from build123d import *

# Parameters (mm, degrees)
F0_W     = 35
F0_H     = 50
F1_DEPTH = 3
F0_W_2   = 38
F0_H_2   = 53
F2_DEPTH = 1.6
F3_DEPTH = 43
F4_R     = 1
F5_W     = 35
F5_H     = 1.5
F6_DEPTH = 41.4


with BuildPart() as f1:
    # F0 (on Top) → F1 (new body)
    with BuildSketch(Plane.XY):
        with Locations((19, 26.5)):
            Rectangle(F0_W, F0_H)
    extrude(amount=-F1_DEPTH)

    # F0 (on Top) → F2 (join)
    with BuildSketch(Plane.XY):
        with Locations((19, 26.5)):
            Rectangle(F0_W_2, F0_H_2)
        with Locations((19, 26.5)):
            Rectangle(F0_W, F0_H, mode=Mode.SUBTRACT)
        with Locations((19, 26.5)):
            Rectangle(F0_W, F0_H)
    extrude(amount=F2_DEPTH)

    # F0 (on Top) → F3 (join)
    with BuildSketch(Plane.XY):
        with Locations((19, 26.5)):
            Rectangle(F0_W_2, F0_H_2)
        with Locations((19, 26.5)):
            Rectangle(F0_W, F0_H, mode=Mode.SUBTRACT)
    extrude(amount=F3_DEPTH)

    # F4
    f4_edges = [f1.edges().sort_by_distance(p)[0] for p in [
        (36.5, 1.5, -1.5),
        (1.5, 1.5, -1.5),
        (1.5, 51.5, -1.5),
        (36.5, 51.5, -1.5),
        (0, 53, 21.5),
        (38, 53, 21.5),
        (0, 0, 21.5),
        (38, 0, 21.5),
    ]]
    fillet(f4_edges, radius=F4_R)

    # F5 (on face) → F6 (join, through all)
    with BuildSketch(Plane.XY.offset(1.6)):
        with Locations((19, 26.5)):
            Rectangle(F5_W, F5_H)
    extrude(amount=F6_DEPTH)


solid = f1.part
Geometry check sheet. Reference: the model listing, model coordinates, mm. A direction names the side the tool comes from. Give positions to 0.01 mm unless a question says otherwise; leave off trailing zeros. Loops run counter-clockwise (first coordinate to the right, second up) from the corner with the lowest first, then second, coordinate; pieces in that order, holes last. Notation, with made-up numbers: M -29.5,7.25 L -18.5,7.25 A19 cw -18.5,19.25 Z; hole C 40.5,6.5 d9. An arc over 180 degrees is marked long. Answer as a JSON object with one key per item and string values. Group by question number.
Item 1: Sectioned sample at C-C on x = 8. Record the boundary of the cut face in (y, z).
Item 2: Sectioned sample at A-A on y = 5.5. Record the boundary of the cut face in (x, z), plus the area to 3 significant figures.
Item 3: Sectioned sample at B-B on z = 24.5. Record the boundary of the cut face in (x, y), plus the area to 3 significant figures.
Item 4: Access from +Z, -Z, +X, -X, +Y, -Y to the whole of each face (thin tool, end or side, straight path). Record for faces 4 (the flat face through (1.5, 26, -1)), 5 (the flat face through (36.5, 39, 22)), 6 (the flat face through (19, 51.5, -1)), 7 (the flat face through (36.5, 26, -1)), 8 (the flat face through (19, 27, 43)).
Item 5: Material ranges on L1, parallel to Y at x = 28, z = 26; L2, parallel to X at y = 38, z = 40.5; L3, parallel to Z at x = 27, y = 36.5, recorded low to high.
Item 6: Mould release check, pull along Y, two halves, no side actions. Record for faces 1 (the flat face through (19, 0, 21)), 2 (the flat face through (19, 25.75, 22)), 3 (the flat face through (1, 27, 0)): pulls with the +Y half, pulls with the -Y half, needs draft (parallel to the pull), parting line crosses it, or undercut.
Item 7: Gauge pin test, flat ends, axial feed: pin 1 (19.5 mm diameter, centred on x = 22.5, y = 37.5, fed in from +Z); pin 2 (1.5 mm diameter, centred on x = 21.5, z = -1, fed in from +Y); pin 3 (2.5 mm diameter, centred on y = 34.5, z = -1.5, fed in from +X). Record the tip position at first contact, or that the pin passes through.
Findings below:
{
 "1": {"outline": "M 0,0 L 1.5,0 L 1.5,-3 L 51.5,-3 L 51.5,0 L 53,0 L 53,43 L 51.5,43 L 51.5,1.6 L 27.25,1.6 L 27.25,43 L 25.75,43 L 25.75,1.6 L 1.5,1.6 L 1.5,43 L 0,43 Z"},
 "2": {"outline": "M 0,0 L 1.5,0 L 1.5,-3 L 36.5,-3 L 36.5,0 L 38,0 L 38,43 L 36.5,43 L 36.5,1.6 L 1.5,1.6 L 1.5,43 L 0,43 Z", "area": "290 mm2"},
 "3": {"outline": "M 0,1 A1 ccw 1,0 L 37,0 A1 ccw 38,1 L 38,52 A1 ccw 37,53 L 1,53 A1 ccw 0,52 Z; hole M 1.5,1.5 L 36.5,1.5 L 36.5,25.75 L 1.5,25.75 Z; hole M 1.5,27.25 L 36.5,27.25 L 36.5,51.5 L 1.5,51.5 Z", "area": "316 mm2"},
 "4": {"face 4": "-Z, -X, +Y, -Y", "face 5": "+Z", "face 6": "-Z, +X, -X, +Y", "face 7": "-Z, +X, +Y, -Y", "face 8": "+Z, +X, -X, +Y, -Y"},
 "5": {"L1": "0 to 1.5, 25.75 to 27.25, 51.5 to 53", "L2": "0 to 1.5, 36.5 to 38", "L3": "-3 to 1.6"},
 "6": {"face 1": "pulls with the -Y half", "face 2": "undercut", "face 3": "needs draft"},
 "7": {"pin 1": "z = 1.6", "pin 2": "y = 51.5", "pin 3": "x = 36.5"}
}
